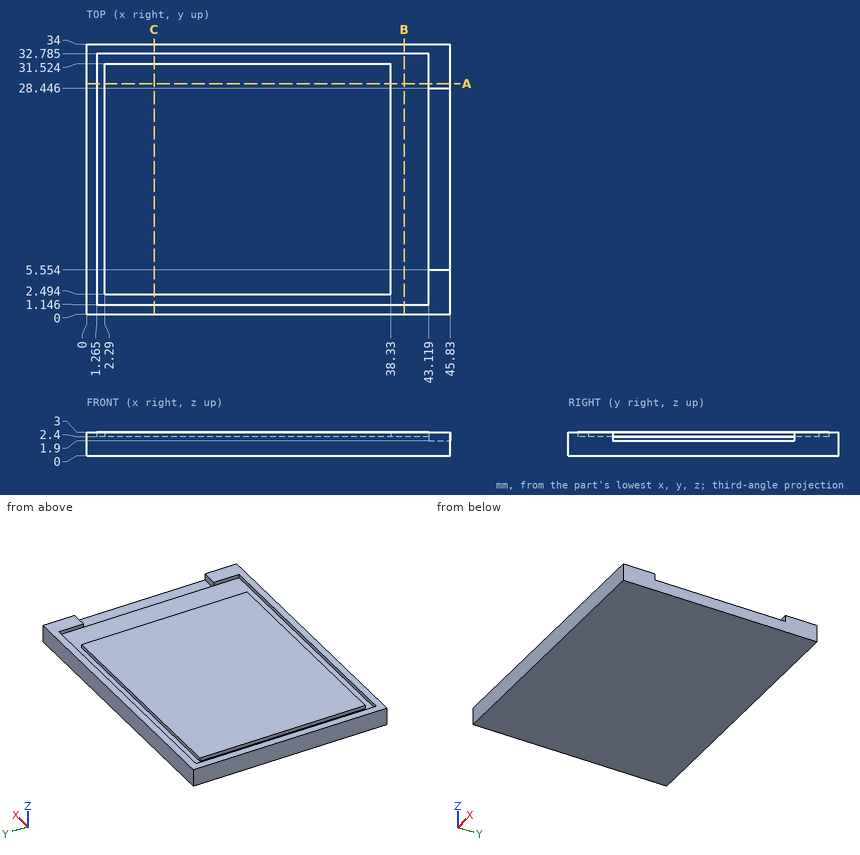
Could you check a few things on this drawing? It's one solid part, dimensions in mm from its lowest x, y, z. Coordinates: 2 decimals unless noted, no trailing zeros. Order: outer loops, then holes, each group sorted by start corner. A loop starts at its lowest first (then second) coordinate and runs counter-clockwise, first axis right, second up. Notation, with made-up numbers: (4.5, 74.5) - (14.5, 74.5) arc R6 cw to (14.5, 81.5) - close; hole circle Ø9 at (-22.5, 10). An arc over 180 degrees is marked (long way). Answer as a JSON object with one key per item and string values. Group by question number.
Q1. Will these pins go through, and if not, where does the flat tip stop? P1, Ø0.8, axis at x = 45, y = 16, coming from the +Z side; P2, Ø0.5, axis at y = 15, z = 2.5, coming from the +X side.
Q2. Imagine slicing it at B-B (x = 40). Please give me the cut outline in (y, z) (1 decimal).
Q3. I need wall thicknesses on line 1 (Y direction, x = 7, z = 2.5) (1 decimal); line 2 (X direction, y = 19.5, z = 2.7) (1 decimal); line 3 (Z direction, x = 40.5, y = 28.5). Which ranges of each line are inside material? Lowest first, please. Write a range as from..to.
Q4. Imagine slicing it at C-C (x = 8.5). Please give me the cut outline in (y, z) (1 decimal), and give its area (3 significant figures).
Q5. Imagine slicing it at A-A (y = 29). Please give me the cut outline in (x, z) (1 decimal), and give its area (3 significant figures).
Determined:
{
 "1": {"P1": "stops at z = 1.9", "P2": "stops at x = 43.12"},
 "2": {"outline": "(0, 0) - (34, 0) - (34, 3) - (32.8, 3) - (32.8, 2.4) - (1.1, 2.4) - (1.1, 3) - (0, 3) - close"},
 "3": {"line 1": "y = 0..1.1, 2.5..31.5, 32.8..34", "line 2": "x = 0..1.3, 2.3..38.3", "line 3": "z = 0..2.4"},
 "4": {"outline": "(0, 0) - (34, 0) - (34, 3) - (32.8, 3) - (32.8, 2.4) - (31.5, 2.4) - (31.5, 3) - (2.5, 3) - (2.5, 2.4) - (1.1, 2.4) - (1.1, 3) - (0, 3) - close", "area": "100 mm2"},
 "5": {"outline": "(0, 0) - (45.8, 0) - (45.8, 3) - (43.1, 3) - (43.1, 2.4) - (38.3, 2.4) - (38.3, 3) - (2.3, 3) - (2.3, 2.4) - (1.3, 2.4) - (1.3, 3) - (0, 3) - close", "area": "134 mm2"}
}
